Can you work these out from the model? Positions are in its coordinate system, mm. A direction names the side the tool comes from. Round coordinates to 2 decimals unless told otherwise and drop trailing zeros. Loops run counter-clockwise (first coordinate to the right, second up) from the corner with the lowest first, then second, coordinate; pieces in that order, holes last.
```python
from build123d import *

# Parameters (mm, degrees)
F1_DEPTH = 2
F3_D     = 1
F5_D     = 4


with BuildPart() as f1:
    # F0 (on Top) → F1 (new body)
    with BuildSketch(Plane.XY):
        with BuildLine():
            Line((1, 3.185364), (1, 7))
            ThreePointArc((1, 7), (0, 8), (-1, 7))
            Line((-1, 7), (-1, 3.185364))
            ThreePointArc((-1, 3.185364), (-1.053313, 3.049412), (-1.18483, 2.985941))
            Line((-1.18483, 2.985941), (-14.146356, 2))
            ThreePointArc((-14.146356, 2), (-16, 0), (-14.146356, -2))
            Line((-14.146356, -2), (-1.18483, -2.985941))
            ThreePointArc((-1.18483, -2.985941), (-1.053313, -3.049412), (-1, -3.185364))
            Line((-1, -3.185364), (-1, -7))
            ThreePointArc((-1, -7), (0, -8), (1, -7))
            Line((1, -7), (1, -3.185364))
            ThreePointArc((1, -3.185364), (1.053313, -3.049412), (1.18483, -2.985941))
            Line((1.18483, -2.985941), (14.146356, -2))
            ThreePointArc((14.146356, -2), (16, 0), (14.146356, 2))
            Line((14.146356, 2), (1.18483, 2.985941))
            ThreePointArc((1.18483, 2.985941), (1.053313, 3.049412), (1, 3.185364))
        make_face()
    extrude(amount=F1_DEPTH)

    # F3 (through all)
    with Locations(Plane.XY.offset(2)):
        with Locations((5, 0), (7, 0), (9, 0), (11, 0), (13, 0), (15, 0), (0, 5), (0, 7), (-5, 0), (-7, 0), (-9, 0), (-11, 0), (-13, 0), (-15, 0), (0, -5), (0, -7)):
            Hole(F3_D / 2)

    # F5 (through all)
    with Locations(Plane.XY.offset(2)):
        with Locations((0, 0)):
            Hole(F5_D / 2)


solid = f1.part
```
(1) If I drill on line 1 (Y direction, x = 0, z = 1.2); line 2 (Y direction, x = -7, z = 1.8); line 3 (X direction, y = -5.25, z = 0.85), over which ranges is the centre line in solid material (lowest first)?
(2) For pin 1 (4 mm diameter, centred on x = 10.5, y = 5.5, fed in from +Z); pin 2 (6 mm diameter, centred on x = 11.5, y = -3, fed in from -Z); pin 3 (0.6 mm diameter, centred on y = -5, z = 1, fed in from -X); pin 4 (1 mm diameter, centred on y = -4, z = 1, fed in from +X), each with a flat end and sliding along its axis, tell me the tip position at first contact or that it passes through.
(3) Suppose I cut it at A-A (x = 0). Write out the boundary of the cut face in (y, z), then the cut area to 3 significant figures.
(4) We'd pull the mould along X, two halves only. Please class faces 1 (the cylindrical face through (0, -8, 1)), 2 (the cylindrical face through (0.065, -4.504, 0.986)), 3 (the flat face through (-1, 5, 1)): released by +X, released by -X, zero draft, split by the parting line, or undercut.
(5) Suppose I cut it at B-B (z = 1.25). Give the number of separate pieces and of enclosed holes in the cut face, then the cut area to 3 significant figures.
(6) Which directions (+Z, -Z, +X, -X, +Y, -Y) give clear straight access to the entire face, cutting with the end or side of a thin tool? Please do faces 4 (the flat face through (1, -5, 1)), 5 (the cylindrical face through (9.5, 0, 1)).
(7) Suppose I cut it at C-C (x = 9). Write out the boundary of the cut face in (y, z), then the cut area to 3 significant figures.
Check result:
1. line 1: y = -8 to -7.5, -6.5 to -5.5, -4.5 to -2, 2 to 4.5, 5.5 to 6.5, 7.5 to 8
1. line 2: y = -2.54 to -0.5, 0.5 to 2.54
1. line 3: x = -1 to -0.43, 0.43 to 1
2. pin 1: passes through
2. pin 2: stops at z = 0
2. pin 3: stops at x = -1
2. pin 4: stops at x = 1
3. outline: (-8, 0) - (-7.5, 0) - (-7.5, 2) - (-8, 2) - close; (-6.5, 0) - (-5.5, 0) - (-5.5, 2) - (-6.5, 2) - close; (-4.5, 0) - (-2, 0) - (-2, 2) - (-4.5, 2) - close; (2, 0) - (4.5, 0) - (4.5, 2) - (2, 2) - close; (5.5, 0) - (6.5, 0) - (6.5, 2) - (5.5, 2) - close; (7.5, 0) - (8, 0) - (8, 2) - (7.5, 2) - close
3. area: 16.0 mm2
4. face 1: split by the parting line
4. face 2: undercut
4. face 3: released by -X
5. separate pieces: 1
5. enclosed holes: 17
5. area: 149 mm2
6. face 4: +Z, -Z, +X, -Y
6. face 5: +Z, -Z
7. outline: (-2.39, 0) - (-0.5, 0) - (-0.5, 2) - (-2.39, 2) - close; (0.5, 0) - (2.39, 0) - (2.39, 2) - (0.5, 2) - close
7. area: 7.57 mm2
